from build123d import *

# Parameters (mm, degrees)
SKETCH1_W           = 93
SKETCH1_H           = 52
BOSS_EXTRUDE1_DEPTH = 25
CUT_EXTRUDE1_DEPTH  = 26
SKETCH3_R           = 4
CUT_EXTRUDE2_DEPTH  = 53


with BuildPart() as part:
    # Sketch1 → Boss-Extrude1 (new body)
    with BuildSketch(Plane.XY):
        Rectangle(SKETCH1_W, SKETCH1_H)
    extrude(amount=BOSS_EXTRUDE1_DEPTH)

    # Sketch2 → Cut-Extrude1 (cut, through all)
    with BuildSketch(Plane(origin=(0, 0, 0), x_dir=(-1, 0, 0), z_dir=(0, 0, -1))):
        with BuildLine():
            Line((0, -10), (20, 10))
            ThreePointArc((20, 10), (20, 13.181980515), (16.818019485, 13.181980515))
            Line((16.818019485, 13.181980515), (0, -3.636038969))
            Line((0, -3.636038969), (-16.818019485, 13.181980515))
            ThreePointArc((-16.818019485, 13.181980515), (-20, 13.181980515), (-20, 10))
            Line((-20, 10), (0, -10))
        make_face()
    extrude(amount=-CUT_EXTRUDE1_DEPTH, mode=Mode.SUBTRACT)

    # Sketch3 → Cut-Extrude2 (cut, through all)
    with BuildSketch(Plane.XZ.offset(26)):
        with Locations((-33, 12.5)):
            Circle(SKETCH3_R)
        with Locations((33, 12.5)):
            Circle(SKETCH3_R)
    extrude(amount=-CUT_EXTRUDE2_DEPTH, mode=Mode.SUBTRACT)


solid = part.part
The model under review builds one solid part; all positions refer to its coordinate system, in mm. A direction names the side the tool comes from. Coordinates: 2 decimals unless noted, no trailing zeros. Write each loop counter-clockwise with the first axis right and the second up, starting at its lowest first coordinate (ties: lowest second). Pieces come first, ordered by that corner, then holes. Notation, with made-up numbers: (-10, 7) - (17, 7) arc R31 cw to (17, 33) - close; hole circle Ø6 at (89, -13.75). An arc over 180 degrees is marked (long way). Answer as CSV lines item,"result".
(1) For line 1 along Z through (x, y) = (33, -10); line 2 along X through (y, z) = (-7, 13.25); line 3 along X through (y, z) = (12, 18.25), list the stretches that pass through material, from the lowest coordinate up. Write a range as [from, to].
Data:
line 1,"z = [0, 8.5], [16.5, 25]"
line 2,"x = [-46.5, -36.93], [-29.07, -3], [3, 29.07], [36.93, 46.5]"
line 3,"x = [-46.5, -20.62], [-15.64, 15.64], [20.62, 46.5]"
(2) We need section A-A (x = -33). Give the boundary of the cut face in (y, z), plus the area to 3 significant figures.
Data:
outline,"(-26, 0) - (26, 0) - (26, 8.5) - (-26, 8.5) - close; (-26, 16.5) - (26, 16.5) - (26, 25) - (-26, 25) - close"
area,"884 mm2"
(3) We need section D-D (z = 7.25). Give the boundary of the cut face in (x, y).
Data:
outline,"(-46.5, -26) - (46.5, -26) - (46.5, 26) - (-46.5, 26) - close; hole (-20, 10) - (0, -10) - (20, 10) arc R2.25 ccw to (16.82, 13.18) - (0, -3.64) - (-16.82, 13.18) arc R2.25 ccw to start"
(4) Clearance check with a flat-ended pin moving along its axis: pin 1 Ø6.5 at (x, z) = (33, 12.5) entering from -Y. State where the tip first meets the part, or that it passes through.
Data:
pin 1,"passes through"
(5) We need section C-C (y = -18.5). Give the boundary of the cut face in (x, z), plus the area to 3 significant figures.
Data:
outline,"(-46.5, 0) - (46.5, 0) - (46.5, 25) - (-46.5, 25) - close; hole circle Ø8 at (-33, 12.5); hole circle Ø8 at (33, 12.5)"
area,"2,220 mm2"
(6) We need section B-B (z = 12.5). Give the boundary of the cut face in (x, y), plus the area to 3 significant figures.
Data:
outline,"(-46.5, -26) - (-37, -26) - (-37, 26) - (-46.5, 26) - close; (-29, -26) - (29, -26) - (29, 26) - (-29, 26) - close; (37, -26) - (46.5, -26) - (46.5, 26) - (37, 26) - close; hole (-20, 10) - (0, -10) - (20, 10) arc R2.25 ccw to (16.82, 13.18) - (0, -3.64) - (-16.82, 13.18) arc R2.25 ccw to start"
area,"3,750 mm2"
(7) Tool access review of faces 1 (the flat face through (-8.527, 4.891, 12.325)), 2 (the flat face through (-1, -26, 12)): name each direction out of +Z, -Z, +X, -X, +Y, -Y from which nothing blocks a thin tool from reaching the whole face with its end or side.
Data:
face 1,"+Z, -Z"
face 2,"+Z, -Z, +X, -X, -Y"
(8) Mouldability with a two-part tool opening along X and no side actions: class faces 3 (the flat face through (46.5, 0, 12)), 4 (the flat face through (-1, 0, 25)), 5 (the cylindrical face through (-35.95, -0.36, 15.2)), 6 (the flat face through (-46.5, 0, 12)) as pulls with the +X half, pulls with the -X half, needs draft (parallel to the pull), parting line crosses it, or undercut.
Data:
face 3,"pulls with the +X half"
face 4,"needs draft"
face 5,"undercut"
face 6,"pulls with the -X half"
